Solid Edge part; units mm, degrees
sketch "Sketch1" plane through (0, 0, 0) normal (0, 0, 1) x (1, 0, 0)
  circle A0 centre (0, 0) radius 101.5
extrude "Protrusion1" add sketch "Sketch1" against normal blind 19
sketch "Sketch2" plane through (0, 0, 0) normal (0, 0, 1) x (1, 0, 0)
  circle A0 centre (0, 0) radius 32
  circle A1 centre (0, 0) radius 16
extrude "ExtrudedProtrusion_2" add sketch "Sketch2" along normal blind 51
sketch "Sketch3" plane through (0, 0, 0) normal (0, 0, 1) x (1, 0, 0)
  circle A0 centre (86, 0) radius 8
extrude "Cutout1" cut sketch "Sketch3" against normal up to vertex (19 mm away)
pattern_circular "Pattern1" count 6 over 360 about axis through (0, 0, 0) along (0, 0, 1) of "Cutout1"
sketch "Sketch4" plane through (0, 0, 0) normal (1, 0, 0) x (0, 1, 0)
  line L0 (32, 51) -> (123.9402, 17.8752)
  line L1 (101.5, -19) -> (117.5, -19)
  line L2 (16, -19) -> (101.5, -19)
  line L3 (16, 0) -> (16, -19)
  line L4 (16, 51) -> (16, 0)
  line L5 (32, 51) -> (16, 51)
  arc A0 (123.9402, 17.8752) -> (117.5, -19) centre (117.5, 0) cw
  circle A1 centre (117.5, 0) radius 6.5
extrude "ExtrudedProtrusion_6" add sketch "Sketch4" along normal mid plane 16
pattern_circular "Pattern3" count 3 over 360 about axis through (0, 0, 0) along (0, 0, 1) of "ExtrudedProtrusion_6"
sketch "Sketch5" plane through (0, 0, 0) normal (0, 0, 1) x (1, 0, 0)
  circle A0 centre (0, 0) radius 16
extrude "ExtrudedCutout_2" cut sketch "Sketch5" against normal blind 19
Work out the finished part from the listing and answer in its coordinate system (mm). A direction names the side the tool comes from. Coordinates: 2 decimals unless noted, no trailing zeros. Order: outer loops, then holes, each group sorted by start corner. A loop starts at its lowest first (then second) coordinate and runs counter-clockwise, first axis right, second up. Notation, with made-up numbers: (82.25, 48) - (108.25, 48) arc R27 ccw to (108.25, 69) - close; hole circle Ø10 at (-13.75, 21). An arc over 180 degrees is marked (long way). Put each result on its own line as item: value. Start each with the question number.
1) For faces 5 (the flat face through (8, 71, 16)), 6 (the flat face through (-8, 71, 16)), 7 (the flat face through (-1, -61, 0)), determine the directions among +Z, -Z, +X, -X, +Y, -Y from which every point of the face is accessible in a straight line to the end or side of a thin tool.
2) Find section A-A (x = 0). Give the vertices of the cut face in (y, z), plus the area to 3 significant figures.
3) For a pull along Z with two mould halves and no side action, classify faces 1 (the cylindrical face through (0, 111, 0)), 2 (the flat face through (22, 10, -19)), 3 (the cylindrical face through (38.7, 67.73, -9.37)), 4 (the cylindrical face through (-104.3, -60.347, 5.767)) as released by +Z, released by -Z, zero draft, split by the parting line, or undercut.
4) Find section B-B (y = 0). Give the vertices of the cut face in (x, z).
5) Find section C-C (y = 73.5). Give the vertices of the cut face in (x, z).
6) Flat-ended cylindrical pins translate along their axes: pin 1 (10 mm diameter, centred on x = 86, z = -11.5, fed in from -Y); pin 2 (8 mm diameter, centred on x = -26.5, z = 36, fed in from -Y); pin 3 (2 mm diameter, centred on x = 2, z = 36, fed in from -Y); pin 4 (18.5 mm diameter, centred on x = 43, y = -74.48, fed in from -Z). Find the tip coordinate at first contact, or state that the pin passes through.
7) Find section D-D (z = 36.5). Give the vertices of the cut face in (x, y).
8) Find the intervals of material crossed by line 1 (Y direction, x = -43, z = -7.25); line 2 (X direction, y = 122, z = 11); line 3 (X direction, y = 5.5, z = 6.5), in increasing order. Write a range as from..to.
Results list:
1. face 5: +Z, +X, +Y
1. face 6: +Z, -X, +Y
1. face 7: +Z, -Y
2. outline: (-101.5, -19) - (-16, -19) - (-16, 51) - (-32, 51) - (-32, 0) - (-101.5, 0) - close; (16, -19) - (117.5, -19) arc R19 ccw to (123.94, 17.88) - (32, 51) - (16, 51) - close; hole circle Ø13 at (117.5, 0)
2. area: 8,670 mm^2
3. face 1: undercut
3. face 2: released by -Z
3. face 3: zero draft
3. face 4: undercut
4. outline: (-101.5, -19) - (-94, -19) - (-94, 0) - (-101.5, 0) - close; (-78, -19) - (-16, -19) - (-16, 51) - (-32, 51) - (-32, 0) - (-78, 0) - close; (16, -19) - (78, -19) - (78, 0) - (32, 0) - (32, 51) - (16, 51) - close; (94, -19) - (101.5, -19) - (101.5, 0) - (94, 0) - close
5. outline: (-70, -19) - (-50.94, -19) - (-50.94, 0) - (-70, 0) - close; (-35.06, -19) - (35.06, -19) - (35.06, 0) - (8, 0) - (8, 36.05) - (-8, 36.05) - (-8, 0) - (-35.06, 0) - close; (50.94, -19) - (70, -19) - (70, 0) - (50.94, 0) - close
6. pin 1: stops at y = -61.78
6. pin 2: stops at y = -26.85
6. pin 3: stops at y = -31.98
6. pin 4: stops at z = -19
7. outline: (-66.57, -29.19) - (-58.57, -43.05) - (-22.83, -22.42) arc R32 ccw to (22.83, -22.42) - (58.57, -43.05) - (66.57, -29.19) - (30.83, -8.56) arc R32 ccw to (8, 30.98) - (8, 72.25) - (-8, 72.25) - (-8, 30.98) arc R32 ccw to (-30.83, -8.56) - close; hole circle Ø32 at (0, 0)
8. line 1: y = -91.94..-82.48, -66.48..66.48, 82.48..91.94
8. line 2: x = -8..8
8. line 3: x = -31.52..-15.02, 15.02..31.52
